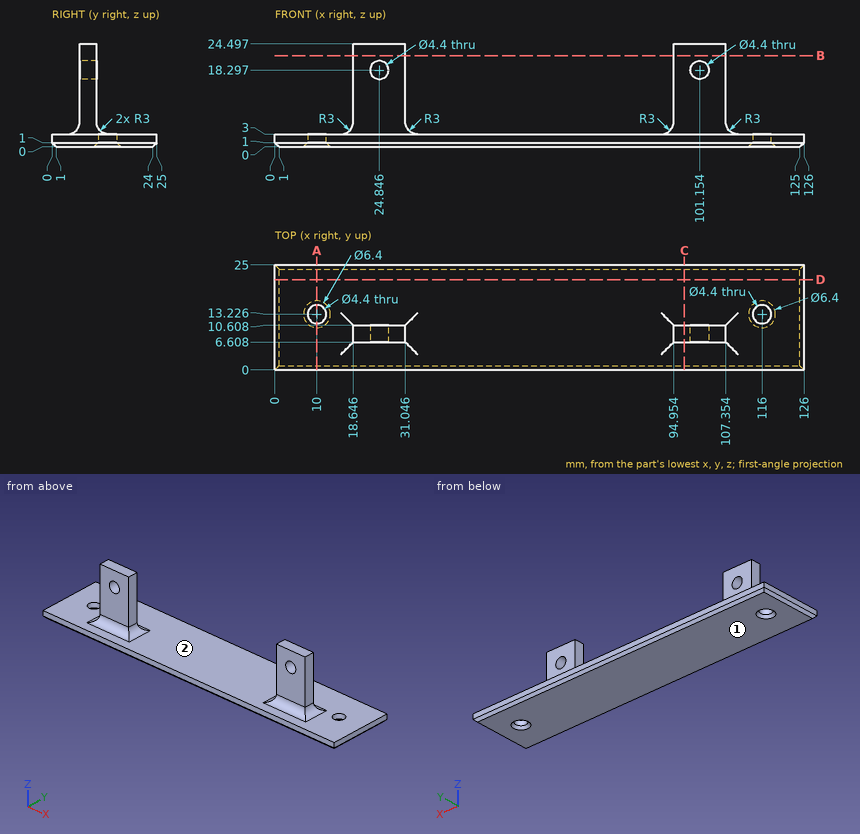
Check sheet for the drawn part. Datum: minimum x, y, z corner. Units: mm. Give positions to 0.01 mm unless a question says otherwise; leave off trailing zeros. Order: outer loops, then holes, each group sorted by start corner. A loop starts at its lowest first (then second) coordinate and runs counter-clockwise, first axis right, second up. Notation, with made-up numbers: (58.5, 14) - (90.5, 14) arc R14 ccw to (90.5, 41) - close; hole circle Ø4 at (9, -31.5). An arc over 180 degrees is marked (long way). Answer as a JSON object with one key per item and string values.
(1) Depth check by flat-ended pin: pin 1 Ø6 at (x, z) = (99, 11.5) entering from -Y; pin 2 Ø5.5 at (x, y) = (116, 13.226) entering from -Z; pin 3 Ø2 at (y, z) = (8.5, 12) entering from +X; pin 4 Ø2.5 at (x, y) = (10, 13.226) entering from -Z. Enter the tip coordinate at first touch or a pass-through.
Report:
{"pin 1": "y = 6.61", "pin 2": "z = 0.45", "pin 3": "x = 107.35", "pin 4": "through"}
(2) Cross-section at B-B (z = 21.75). Record the cut outline in (x, y), then the cut area to 3 significant figures.
Report:
{"outline": "(18.65, 6.61) - (31.05, 6.61) - (31.05, 10.61) - (18.65, 10.61) - close; (94.95, 6.61) - (107.35, 6.61) - (107.35, 10.61) - (94.95, 10.61) - close", "area": "99.2 mm^2"}
(3) Draft check along X on the marked faces 1 and 2. Enter one of: released by +X, released by -X, zero draft, split by the parting line, or undercut.
Report:
{"face 1": "zero draft", "face 2": "undercut"}
(4) Cross-section at D-D (y = 21.5). Record the cut outline in (x, z), then the cut area to 3 significant figures.
Report:
{"outline": "(0, 1) - (1, 0) - (125, 0) - (126, 1) - (126, 3) - (0, 3) - close", "area": "377 mm^2"}
(5) Cross-section at A-A (x = 10). Record the cut outline in (y, z), then the cut area to 3 significant figures.
Report:
{"outline": "(0, 1) - (1, 0) - (10.03, 0) - (11.03, 1) - (11.03, 3) - (0, 3) - close; (15.43, 1) - (16.43, 0) - (24, 0) - (25, 1) - (25, 3) - (15.43, 3) - close", "area": "59.8 mm^2"}
(6) Material ranges on line 1 (Y direction, x = 116, z = 2.45); line 2 (X direction, y = 7.75, z = 6); line 3 (X direction, y = 10, z = 17.75), recorded low to high.
Report:
{"line 1": "0 to 11.03, 15.43 to 25", "line 2": "18.65 to 31.05, 94.95 to 107.35", "line 3": "18.65 to 22.72, 26.98 to 31.05, 94.95 to 99.02, 103.28 to 107.35"}
(7) Cross-section at C-C (x = 97.5). Record the cut outline in (y, z).
Report:
{"outline": "(0, 1) - (1, 0) - (24, 0) - (25, 1) - (25, 3) - (13.61, 3) arc R3 cw to (10.61, 6) - (10.61, 24.5) - (6.61, 24.5) - (6.61, 6) arc R3 cw to (3.61, 3) - (0, 3) - close"}
